```python
from build123d import *

# Parameters (mm, degrees)
SKETCH1_R           = 1.6
BOSS_EXTRUDE1_DEPTH = 3.75


with BuildPart() as part:
    # Sketch1 → Boss-Extrude1 (new body)
    with BuildSketch(Plane.XY):
        with BuildLine():
            Line((0, -22.114150905), (0, -5))
            ThreePointArc((0, -5), (3.535533906, 3.535533906), (-5, 0))
            Line((-5, 0), (-5.114562262, -22.904716871))
            Line((-5.114562262, -22.904716871), (-12.863985131, -26.761912172))
            ThreePointArc((-12.863985131, -26.761912172), (-14.071191727, -29.928476691), (-11.013170041, -31.388949897))
            Line((-11.013170041, -31.388949897), (-0.755279555, -28.225082361))
            ThreePointArc((-0.755279555, -28.225082361), (1.599513904, -25.413982613), (0, -22.114150905))
        make_face()
        Circle(SKETCH1_R, mode=Mode.SUBTRACT)
        with Locations((-1.75, -25)):
            Circle(SKETCH1_R, mode=Mode.SUBTRACT)
        with Locations((-11.75, -29)):
            Circle(SKETCH1_R, mode=Mode.SUBTRACT)
    extrude(amount=BOSS_EXTRUDE1_DEPTH)


solid = part.part
```
The model under review builds one solid part; all positions refer to its coordinate system, in mm. A direction names the side the tool comes from. Round coordinates to 2 decimals unless told otherwise and drop trailing zeros. Write each loop counter-clockwise with the first axis right and the second up, starting at its lowest first coordinate (ties: lowest second). Pieces come first, ordered by that corner, then holes.
(1) Mouldability with a two-part tool opening along Y and no side actions: class faces 1 (the flat face through (-5.96, -29.83, 1.85)), 2 (the cylindrical face through (-1.958, -23.414, 1.849)), 3 (the flat face through (-8.94, -24.81, 1.85)) as +Y half, -Y half, draft (parallel to the pull), parting line (faces both ways), or undercut.
(2) Wall thickness on L1, parallel to Y at x = 1, z = 1.8; L2, parallel to X at y = -24.5, z = 3.45; L3, parallel to Y at x = -11.75, z = 1.75: over which ranges is each line inside the solid? List them lowest first.
(3) We need section B-B on y = -25. Give the boundary of the cut face in (x, z) (3 decimals).
(4) Insertion check: pin 1 (1.5 mm diameter, centred on y = -3, z = 2.5, fed in from +X); pin 2 (2.5 mm diameter, centred on x = -11.75, y = -29, fed in from -Z); pin 3 (1.5 mm diameter, centred on y = -24.5, z = 1.5, fed in from -X). Each pin has a flat end and moves straight along its axis. Give the tip position at first contact, or say it passes through.
(5) We need section C-C on x = -11.75. Give the boundary of the cut face in (y, z), and give its area (3 significant figures).
(6) Machinability: for faces 4 (the flat face through (0, -14, 2)), 5 (the cylindrical face through (-13, -28, 2)), which of the approach directions +Z, -Z, +X, -X, +Y, -Y give a long, thin tool a straight path to every point of the face, cutting with its end or side? Answer none if there is none.
(7) We need section A-A on z = 2.15. Give the boundary of the cut face in (x, y) (3 decimals), and give its area (3 significant figures).
(8) We need section D-D on x = -4.5. Give the boundary of the cut face in (y, z).
Findings below:
1. face 1: -Y half
1. face 2: undercut
1. face 3: +Y half
2. L1: y = -26.96 to -23.04, -4.9 to -1.25, 1.25 to 4.9
2. L2: x = -8.32 to -3.27, -0.23 to 1.59
2. L3: y = -31.5 to -30.6, -27.4 to -26.21
3. outline: (-9.324, 0) - (-3.35, 0) - (-3.35, 3.75) - (-9.324, 3.75) - close; (-0.15, 0) - (1.625, 0) - (1.625, 3.75) - (-0.15, 3.75) - close
4. pin 1: stops at x = 4.47
4. pin 2: passes through
4. pin 3: stops at x = -9.83
5. outline: (-31.5, 0) - (-30.6, 0) - (-30.6, 3.75) - (-31.5, 3.75) - close; (-27.4, 0) - (-26.21, 0) - (-26.21, 3.75) - (-27.4, 3.75) - close
5. area: 7.85 mm2
6. face 4: +Z, -Z, +X
6. face 5: +Z, -Z
7. outline: (-12.864, -26.762) arc R2.5 ccw to (-11.013, -31.389) - (-0.755, -28.225) arc R3.375 ccw to (0, -22.114) - (0, -5) arc R5 ccw (long way) to (-5, 0) - (-5.115, -22.905) - close; hole circle Ø3.2 at (-11.75, -29); hole circle Ø3.2 at (-1.75, -25); hole circle Ø3.2 at (0, 0)
7. area: 237 mm2
8. outline: (-29.38, 0) - (2.18, 0) - (2.18, 3.75) - (-29.38, 3.75) - close
